Build history of the part. All positions in model axes, mm. A direction names the side the tool comes from. Round coordinates to 2 decimals unless told otherwise and drop trailing zeros. Write each loop counter-clockwise with the first axis right and the second up, starting at its lowest first coordinate (ties: lowest second). Pieces come first, ordered by that corner, then holes. Notation, with made-up numbers: M 45.5,-11.75 L 97.5,-11.75 A24 cw 97.5,16.25 Z; hole C 57,47 d5. An arc over 180 degrees is marked long. One line per item, written item: value. Start each with the question number.
```python
from build123d import *

# Parameters (mm, degrees)
CROQUIS1_R                     = 12.5
CROQUIS1_R_2                   = 4.5
CROQUIS1_R_3                   = 2.9
SALIENTE_EXTRUIR1_DEPTH        = 2
CROQUIS1_3_R                   = 4.5
CROQUIS1_3_R_2                 = 2.9
SALIENTE_EXTRUIR2_DEPTH        = 4
TALADRO_DE_MARGEN_PARA_M1_61_D = 1.8


with BuildPart() as part:
    # Croquis1 → Saliente-Extruir1 (new body)
    # profile 1 of 3: a face of its own
    with BuildSketch(Plane(origin=(0, 0, 0), x_dir=(1, 0, 0), z_dir=(0, 1, 0))):
        with Locations(Location((0, 0, 0), (0, 0, 270))):
            Circle(CROQUIS1_R)
        Circle(CROQUIS1_R_2, mode=Mode.SUBTRACT)
    # profile 2 of 3: a face of its own
    with BuildSketch(Plane(origin=(0, 0, 0), x_dir=(1, 0, 0), z_dir=(0, 1, 0))):
        Circle(CROQUIS1_R_2)
        Circle(CROQUIS1_R_3, mode=Mode.SUBTRACT)
    # profile 3 of 3: a face of its own
    with BuildSketch(Plane(origin=(0, 0, 0), x_dir=(1, 0, 0), z_dir=(0, 1, 0))):
        Circle(CROQUIS1_R_3)
    extrude(amount=SALIENTE_EXTRUIR1_DEPTH)

    # Croquis1<3> → Saliente-Extruir2 (add)
    with BuildSketch(Plane(origin=(0, 0, 0), x_dir=(1, 0, 0), z_dir=(0, 1, 0))):
        with Locations(Location((0, 0, 0), (0, 0, 270))):
            Circle(CROQUIS1_3_R)
        with Locations(Location((0, 0, 0), (0, 0, 270))):
            Circle(CROQUIS1_3_R_2, mode=Mode.SUBTRACT)
    extrude(amount=-SALIENTE_EXTRUIR2_DEPTH)

    # Taladro de margen para M1.61 (through all)
    with Locations(Plane.ZX.offset(2)):
        with Locations((0, 0), (-7.5, 0), (0, 7.5), (7.5, 0), (0, -7.5)):
            Hole(TALADRO_DE_MARGEN_PARA_M1_61_D / 2)


solid = part.part
```
Item 1: Cut at B-B, the plane y = 0.95. Write the cut outline in (x, z).
Item 2: Cut at D-D, the plane z = 0. Write the cut outline in (x, y).
Item 3: Cut at A-A, the plane x = 0. Write the cut outline in (y, z), plus the area to 3 significant figures.
Item 4: Cut at C-C, the plane z = 7.5. Write the cut outline in (x, y).
Item 5: Which spindle directions (+Z, -Z, +X, -X, +Y, -Y) get a long thin tool onto all of the face, cutting with end or side? Do faces 1 (the cylindrical face through (0.27, 0.99, 6.64)), 2 (the cylindrical face through (1.352, -1.972, 4.292)). Say none if no direction does.
Item 6: Drill centre lines: line 1 (X direction, y = 0.65, z = 0); line 2 (Y direction, x = -4.25, z = 10); line 3 (Z direction, x = -0.5, y = -2.65). Where is each one in solid material? Low to high.
Item 7: Drop flat-ended pins along their axis: pin 1 (1.5 mm diameter, centred on y = -2, z = 9.5, fed in from +X); pin 2 (2.5 mm diameter, centred on x = 0, z = -7.5, fed in from -Y); pin 3 (1 mm diameter, centred on x = -0.5, y = -1, fed in from -Z); pin 4 (3 mm diameter, centred on x = -6, y = 0, fed in from -Z). Give the stop position or say it passes through.
Item 8: Two-plate mould, pull along Z, no slides. Class faces 3 (the cylindrical face through (3.755, 0.986, 11.923)), 4 (the cylindrical face through (8.39, 0.99, 0.12)), 5 (the flat face through (0, 0, 5)), 6 (the flat face through (1, 0, -1)): pulls with the +Z half, pulls with the -Z half, needs draft (parallel to the pull), parting line crosses it, or undercut.
Computed values:
1. outline: C 0,0 d25; hole C -7.5,0 d1.8; hole C 0,-7.5 d1.8; hole C 0,0 d1.8; hole C 0,7.5 d1.8; hole C 7.5,0 d1.8
2. outline: M -12.5,0 L -8.4,0 L -8.4,2 L -12.5,2 Z; M -6.6,0 L -4.5,0 L -4.5,-4 L -2.9,-4 L -2.9,0 L -0.9,0 L -0.9,2 L -6.6,2 Z; M 0.9,0 L 2.9,0 L 2.9,-4 L 4.5,-4 L 4.5,0 L 6.6,0 L 6.6,2 L 0.9,2 Z; M 8.4,0 L 12.5,0 L 12.5,2 L 8.4,2 Z
3. outline: M -4,-4.5 L 0,-4.5 L 0,-6.6 L 2,-6.6 L 2,-0.9 L 0,-0.9 L 0,-2.9 L -4,-2.9 Z; M -4,2.9 L 0,2.9 L 0,0.9 L 2,0.9 L 2,6.6 L 0,6.6 L 0,4.5 L -4,4.5 Z; M 0,-12.5 L 2,-12.5 L 2,-8.4 L 0,-8.4 Z; M 0,8.4 L 2,8.4 L 2,12.5 L 0,12.5 Z
3. area: 52.0 mm2
4. outline: M -10,0 L -0.9,0 L -0.9,2 L -10,2 Z; M 0.9,0 L 10,0 L 10,2 L 0.9,2 Z
5. face 1: +Y, -Y
5. face 2: -Y
6. line 1: x = -12.5 to -8.4, -6.6 to -0.9, 0.9 to 6.6, 8.4 to 12.5
6. line 2: y = 0 to 2
6. line 3: z = -4.47 to -2.86, 2.86 to 4.47
7. pin 1: passes through
7. pin 2: stops at y = 0
7. pin 3: stops at z = -4.5
7. pin 4: stops at z = -11.66
8. face 3: parting line crosses it
8. face 4: undercut
8. face 5: needs draft
8. face 6: undercut
